```python
from build123d import *

# Parameters (mm, degrees)
F0_W     = 76.2
F0_H     = 63.5
F0_R     = 3.175
F1_DEPTH = 19.05
F2_R     = 4.7625
F3_DEPTH = 6.35
F4_R     = 4.7625
F5_DEPTH = 12.701


with BuildPart() as f1:
    # F0 (on Top) → F1 (new body)
    with BuildSketch(Plane.XY):
        with Locations((38.1, 31.75)):
            Rectangle(F0_W, F0_H)
        with Locations((9.525, 9.525)):
            Circle(F0_R, mode=Mode.SUBTRACT)
        with Locations((66.675, 9.525)):
            Circle(F0_R, mode=Mode.SUBTRACT)
        with Locations((9.525, 53.975)):
            Circle(F0_R, mode=Mode.SUBTRACT)
        with Locations((66.675, 53.975)):
            Circle(F0_R, mode=Mode.SUBTRACT)
    extrude(amount=F1_DEPTH)

    # F2 (on face) → F3 (cut)
    with BuildSketch(Plane.XY.offset(19.05)):
        with BuildLine():
            Line((19.05, 63.5), (19.05, 0))
            Line((19.05, 0), (57.15, 0))
            Line((57.15, 0), (57.15, 33.02))
            ThreePointArc((57.15, 33.02), (64.77, 40.64), (57.15, 48.26))
            Line((57.15, 48.26), (49.53, 48.26))
            Line((49.53, 48.26), (34.29, 63.5))
            Line((34.29, 63.5), (19.05, 63.5))
        make_face()
        with Locations((38.1, 32.749232)):
            Circle(F2_R, mode=Mode.SUBTRACT)
        with Locations((38.1, 32.749232)):
            Circle(F2_R)
    extrude(amount=-F3_DEPTH, mode=Mode.SUBTRACT)

    # F4 (on face) → F5 (cut, through all)
    with BuildSketch(Plane.XY.offset(12.7)):
        with Locations((38.1, 32.749232)):
            Circle(F4_R)
    extrude(amount=-F5_DEPTH, mode=Mode.SUBTRACT)


solid = f1.part
```
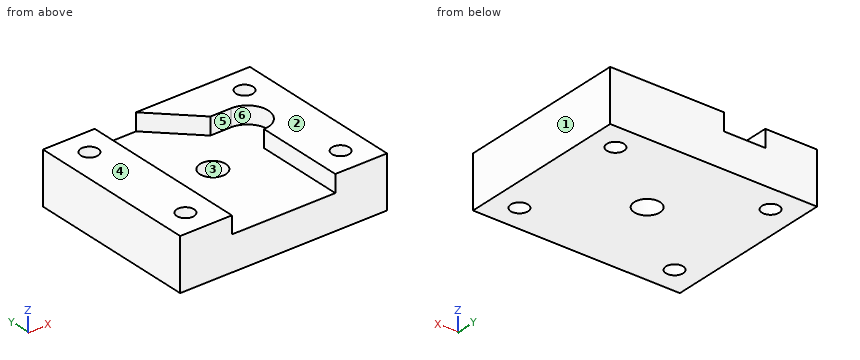
Read the model definition and answer for the solid it produces. Units are mm, in the model's axes. Face numbers are marked on the shaded views. A direction names the side the tool comes from. Give positions to 0.01 mm unless a question says otherwise; leave off trailing zeros. Loops run counter-clockwise (first coordinate to the right, second up) from the corner with the lowest first, then second, coordinate; pieces in that order, holes last.
Item 1: The mould has two halves that part along X. Classify the marked faces 1, 2 and 3: released by +X, released by -X, zero draft, split by the parting line, or undercut.
Item 2: For the marked faces 4, 5 and 6, determine the directions among +Z, -Z, +X, -X, +Y, -Y from which every point of the face is accessible in a straight line to the end or side of a thin tool.
Item 3: The part is cut by section C-C (y = 40.64). Write down the section's boundary in (x, z), and give its area (3 significant figures).
Item 4: The part is cut by section A-A (x = 38.1). Write down the section's boundary in (y, z), and give its area (3 significant figures).
Item 5: The part is cut by section D-D (x = 47.5). Write down the section's boundary in (y, z).
Item 6: Find the intervals of material crossed by line 1 along Y through (x, z) = (9.5, 4.75); line 2 along Y through (x, z) = (38.1, 7.5); line 3 along X through (y, z) = (28, 13.5), in increasing order.
Item 7: Each of these flat-tipped pins is pushed along its axis until it touches: pin 1 Ø4 at (x, y) = (48.5, 22) entering from +Z; pin 2 Ø5 at (x, z) = (54, 17) entering from -Y; pin 3 Ø5.5 at (x, y) = (9.525, 53.975) entering from -Z (1 decimal); pin 4 Ø10 at (x, y) = (66.675, 9.525) entering from +Z. Where does it stop, or does it pass through?
Item 8: The part is cut by section B-B (z = 16.5). Write down the section's boundary in (x, y) (3 decimals), and give its area (3 significant figures).
Taken from the geometry:
1. face 1: released by +X
1. face 2: zero draft
1. face 3: undercut
2. face 4: +Z, +X, -X, +Y, -Y
2. face 5: +Z, -Y
2. face 6: +Z
3. outline: (0, 0) - (76.2, 0) - (76.2, 19.05) - (64.77, 19.05) - (64.77, 12.7) - (19.05, 12.7) - (19.05, 19.05) - (0, 19.05) - close
3. area: 1,160 mm2
4. outline: (0, 0) - (27.99, 0) - (27.99, 12.7) - (0, 12.7) - close; (37.51, 0) - (63.5, 0) - (63.5, 19.05) - (59.69, 19.05) - (59.69, 12.7) - (37.51, 12.7) - close
4. area: 710 mm2
5. outline: (0, 0) - (63.5, 0) - (63.5, 19.05) - (50.29, 19.05) - (50.29, 12.7) - (0, 12.7) - close
6. line 1: y = 0 to 6.35, 12.7 to 50.8, 57.15 to 63.5
6. line 2: y = 0 to 27.99, 37.51 to 63.5
6. line 3: x = 0 to 19.05, 57.15 to 76.2
7. pin 1: stops at z = 12.7
7. pin 2: stops at y = 48.26
7. pin 3: passes through
7. pin 4: stops at z = 19.05
8. outline: (0, 0) - (19.05, 0) - (19.05, 63.5) - (0, 63.5) - close; (34.29, 63.5) - (49.53, 48.26) - (57.15, 48.26) arc R7.62 cw to (57.15, 33.02) - (57.15, 0) - (76.2, 0) - (76.2, 63.5) - close; hole circle Ø6.35 at (9.525, 9.525); hole circle Ø6.35 at (9.525, 53.975); hole circle Ø6.35 at (66.675, 9.525); hole circle Ø6.35 at (66.675, 53.975)
8. area: 2,430 mm2
